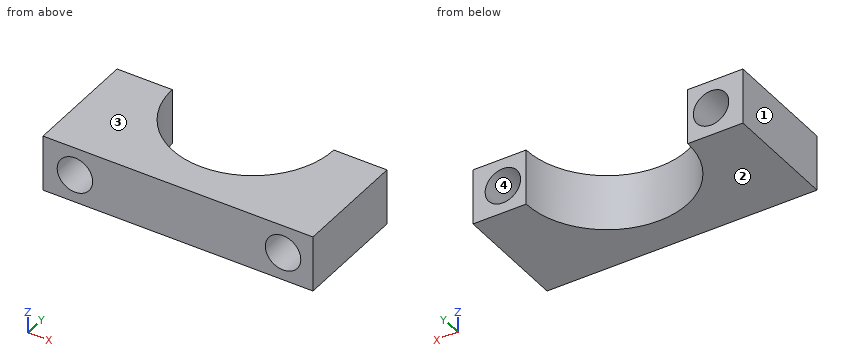
from build123d import *

# Parameters (mm, degrees)
BOSS_EXTRUDE1_DEPTH = 5.52
SKETCH2_R           = 1.75
CUT_EXTRUDE1_DEPTH  = 30.499106766


with BuildPart() as part:
    # Sketch1 → Boss-Extrude1 (new body)
    with BuildSketch(Plane.XY):
        with BuildLine():
            Line((21.4, 11.38), (26.65, 11.38))
            Line((26.65, 11.38), (26.65, 0))
            Line((26.65, 0), (0, 0))
            Line((0, 0), (0, 11.38))
            Line((0, 11.38), (5.45, 11.38))
            ThreePointArc((5.45, 11.38), (13.425, 3.405), (21.4, 11.38))
        make_face()
    extrude(amount=BOSS_EXTRUDE1_DEPTH)

    # Sketch2 → Cut-Extrude1 (cut, through all)
    with BuildSketch(Plane(origin=(0, 11.38, 0), x_dir=(1, 0, 0), z_dir=(0, 1, 0))):
        with Locations(Location((3.15, -2.76, 0), (0, 0, 270))):
            Circle(SKETCH2_R)
        with Locations(Location((23.7, -2.76, 0), (0, 0, 90))):
            Circle(SKETCH2_R)
    extrude(amount=-CUT_EXTRUDE1_DEPTH, mode=Mode.SUBTRACT)


solid = part.part
Source: CAD feature listing. Evaluate the final solid. Frame: model axes, mm. Face numbers are marked on the shaded views. Give positions to 0.01 mm unless a question says otherwise; leave off trailing zeros. Write each loop counter-clockwise with the first axis right and the second up, starting at its lowest first coordinate (ties: lowest second). Pieces come first, ordered by that corner, then holes. Notation, with made-up numbers: M 29.25,74.25 L 81.25,74.25 A19 cw 81.25,88.25 Z; hole C 76,3.5 d7. An arc over 180 degrees is marked long. Return JSON: item names as keys, results as strings. Group by question number.
1) Cut plane C-C, the plane y = 8.25. Output: boundary loops of the cut face in (x, z), then the cut area to 3 significant figures.
2) Draft query along Z for the marked faces 1, 2, 3 and 4. Return one class per face: released by +Z, released by -Z, zero draft, split by the parting line, or undercut.
3) Ray query, L1, parallel to X at y = 2.5, z = 2.76; L2, parallel to X at y = 6.75, z = 2.76; L3, parallel to X at y = 9, z = 2.76. Return the intervals inside material, ascending.
4) Cut plane D-D, the plane y = 2.25. Output: boundary loops of the cut face in (x, z), then the cut area to 3 significant figures.
5) Cut plane B-B, the plane x = 23.7. Output: boundary loops of the cut face in (y, z).
6) Cut plane A-A, the plane z = 2.76. Output: boundary loops of the cut face in (x, y) (3 decimals).
7) First-contact query: pin 1 Ø1.5 at (x, z) = (8.5, 2) entering from +Y; pin 2 Ø1 at (x, z) = (12.5, 4) entering from +Y; pin 3 Ø3 at (x, z) = (23.7, 2.76) entering from -Y. Flat tips, straight axial feed; report the tip coordinate or a pass-through.
Data:
{
 "1": {"outline": "M 0,0 L 6.09,0 L 6.09,5.52 L 0,5.52 Z; M 20.76,0 L 26.65,0 L 26.65,5.52 L 20.76,5.52 Z; hole C 3.15,2.76 d3.5; hole C 23.7,2.76 d3.5", "area": "46.9 mm²"},
 "2": {"face 1": "zero draft", "face 2": "released by -Z", "face 3": "released by +Z", "face 4": "undercut"},
 "3": {"L1": "x = 0 to 1.4, 4.9 to 21.95, 25.45 to 26.65", "L2": "x = 0 to 1.4, 4.9 to 6.93, 19.92 to 21.95, 25.45 to 26.65", "L3": "x = 0 to 1.4, 4.9 to 5.81, 21.04 to 21.95, 25.45 to 26.65"},
 "4": {"outline": "M 0,0 L 26.65,0 L 26.65,5.52 L 0,5.52 Z; hole C 3.15,2.76 d3.5; hole C 23.7,2.76 d3.5", "area": "128 mm²"},
 "5": {"outline": "M 0,0 L 11.38,0 L 11.38,1.01 L 0,1.01 Z; M 0,4.51 L 11.38,4.51 L 11.38,5.52 L 0,5.52 Z"},
 "6": {"outline": "M 0,0 L 1.4,0 L 1.4,11.38 L 0,11.38 Z; M 4.9,0 L 21.95,0 L 21.95,11.38 L 21.4,11.38 A7.975 cw 5.45,11.38 L 4.9,11.38 Z; M 25.45,0 L 26.65,0 L 26.65,11.38 L 25.45,11.38 Z"},
 "7": {"pin 1": "stops at y = 5.78", "pin 2": "stops at y = 3.53", "pin 3": "passes through"}
}
